```python
from build123d import *

# Parameters (mm, degrees)
F0_W     = 812.8
F0_H     = 101.6
F1_DEPTH = 12
F3_DEPTH = 508
F4_R     = 3.96875
F5_DEPTH = 9.525
F6_R     = 3.96875
F7_DEPTH = 9.525


# Not quite as in the source:
# - a length typed as a fraction of an inch, garbled in the dataset ("3 / 203.2 mm" for 3/8 in), is restored


with BuildPart() as f1:
    # F0 (on Top) → F1 (new body)
    with BuildSketch(Plane.XY):
        with Locations((406.4, 50.8)):
            Rectangle(F0_W, F0_H)
    extrude(amount=F1_DEPTH)

    # F2 (on face) → F3 (join)
    with BuildSketch(Plane(origin=(0, 0, 0), x_dir=(1, 0, 0), z_dir=(0, 0, -1))):
        Polygon((12, 0), (0, 0), (0, -101.6), (12, -101.6), (12, -52.2239353538), (800.8, -52.2239353538), (800.8, -101.6), (812.8, -101.6), (812.8, 0), (800.8, 0), (800.8, -40.2239353538), (12, -40.2239353538), align=None)
    extrude(amount=F3_DEPTH)

    # F4 (on face) → F5 (cut)
    with BuildSketch(Plane.YZ.offset(812.8)):
        with Locations((50.8, -172.15)):
            Circle(F4_R)
        with Locations((50.8, -229.3)):
            Circle(F4_R)
        with Locations((50.8, -394.4)):
            Circle(F4_R)
    extrude(amount=-F5_DEPTH, mode=Mode.SUBTRACT)

    # F6 (on face) → F7 (cut)
    with BuildSketch(Plane(origin=(0, 0, 0), x_dir=(0, -1, 0), z_dir=(-1, 0, 0))):
        with Locations((-50.8, -172.15)):
            Circle(F6_R)
        with Locations((-50.8, -229.3)):
            Circle(F6_R)
        with Locations((-50.8, -394.4)):
            Circle(F6_R)
    extrude(amount=-F7_DEPTH, mode=Mode.SUBTRACT)


solid = f1.part
```
Input: part model. Units: mm. Frame: model coordinates. A direction names the side the tool comes from. Give positions to 0.01 mm unless a question says otherwise; leave off trailing zeros. Order: outer loops, then holes, each group sorted by start corner. A loop starts at its lowest first (then second) coordinate and runs counter-clockwise, first axis right, second up.
1. Cut plane B-B (x = 256.5). Return loops of the section in (y, z), and give its area (3 significant figures).
Computed:
outline: (0, 0) - (40.22, 0) - (40.22, -508) - (52.22, -508) - (52.22, 0) - (101.6, 0) - (101.6, 12) - (0, 12) - close
area: 7,320 mm2
2. Pin query (flat end, axial travel): pin 1 Ø8.5 at (y, z) = (49.5, -228.5) entering from -X; pin 2 Ø1 at (x, z) = (418, -74.5) entering from -Y; pin 3 Ø10 at (x, z) = (168.5, -318.5) entering from +Y; pin 4 Ø2 at (x, y) = (639, 27.5) entering from -Z. Return the tip coordinate at first contact, or that it passes through.
Computed:
pin 1: stops at x = 0
pin 2: stops at y = 40.22
pin 3: stops at y = 52.22
pin 4: stops at z = 0
3. Line query: probe 1 along Z at (x, y) = (7, 50.8); probe 2 along Z at (x, y) = (808, 50); probe 3 along X at (y, z) = (18, -295). Output: solid intervals per line, ascending.
Computed:
probe 1: z = -508 to -398.37, -390.43 to -233.27, -225.33 to -176.12, -168.18 to 12
probe 2: z = -508 to -398.29, -390.51 to -233.19, -225.41 to -176.04, -168.26 to 12
probe 3: x = 0 to 12, 800.8 to 812.8
4. Cut plane C-C (y = 25.5). Return loops of the section in (x, z), and give its area (3 significant figures).
Computed:
outline: (0, -508) - (12, -508) - (12, 0) - (800.8, 0) - (800.8, -508) - (812.8, -508) - (812.8, 12) - (0, 12) - close
area: 21,900 mm2
5. Cut plane A-A (z = -426.5). Return loops of the section in (x, y).
Computed:
outline: (0, 0) - (12, 0) - (12, 40.22) - (800.8, 40.22) - (800.8, 0) - (812.8, 0) - (812.8, 101.6) - (800.8, 101.6) - (800.8, 52.22) - (12, 52.22) - (12, 101.6) - (0, 101.6) - close
6. Draft query along X for faces 1 (the face through (800.8, 20, -250)), 2 (the face through (12, 20, -250)), 3 (the face through (405, 47, -508)), 4 (the face through (812.8, 50, -252)). Return one class per face: released by +X, released by -X, zero draft, split by the parting line, or undercut.
Computed:
face 1: undercut
face 2: undercut
face 3: zero draft
face 4: released by +X
7. Set-up query: faces 5 (the face through (408, 0, 4)), 6 (the face through (401, 20, 0)), 7 (the face through (401, 52.224, -250)). Return all of +Z, -Z, +X, -X, +Y, -Y with unobstructed straight access to the full face (end or side cutting, diameter ignored); none if empty.
Computed:
face 5: +Z, -Z, +X, -X, -Y
face 6: -Z, -Y
face 7: -Z, +Y
